from build123d import *

# Parameters (mm, degrees)
SKETCH2_R           = 1.55
CUT_EXTRUDE1_DEPTH  = 33.995567884
SKETCH3_R           = 1.45
BOSS_EXTRUDE1_DEPTH = 1.27
CHAMFER1_SIZE       = 2.54


with BuildPart() as part:
    # Sketch1 → Revolve1 (revolve)
    with BuildSketch(Plane(origin=(0, 0, 0), x_dir=(0, 0, -1), z_dir=(1, 0, 0))):
        Polygon((0, 0), (0, -6.35), (-4.975, -6.35), (-4.975, 0), (-19.05, 0), (-19.05, 12.7), (0, 12.7), align=None)
    revolve(axis=Axis((0, 12.7, 0), (0, -1, 0)))

    # Sketch2 → Cut-Extrude1 (cut, through all)
    with BuildSketch(Plane(origin=(0, 12.7, 0), x_dir=(1, 0, 0), z_dir=(0, 1, 0))):
        with Locations(Location((0, 9, 0), (0, 0, 270))):
            Circle(SKETCH2_R)
        with Locations(Location((0, -9, 0), (0, 0, 270))):
            Circle(SKETCH2_R)
        with Locations(Location((9, 0, 0), (0, 0, 270))):
            Circle(SKETCH2_R)
        with Locations(Location((-9, 0, 0), (0, 0, 270))):
            Circle(SKETCH2_R)
    extrude(amount=-CUT_EXTRUDE1_DEPTH, mode=Mode.SUBTRACT)

    # Sketch3 → Boss-Extrude1 (add)
    with BuildSketch(Plane.XZ):
        with Locations(Location((-5.08, -5.08, 0), (0, 0, 270))):
            Circle(SKETCH3_R)
        with Locations(Location((-5.08, 5.08, 0), (0, 0, 270))):
            Circle(SKETCH3_R)
        with Locations(Location((5.08, 5.08, 0), (0, 0, 270))):
            Circle(SKETCH3_R)
        with Locations(Location((5.08, -5.08, 0), (0, 0, 270))):
            Circle(SKETCH3_R)
    extrude(amount=BOSS_EXTRUDE1_DEPTH)

    # Chamfer1
    chamfer1_edges = [part.edges().sort_by_distance(p)[0] for p in [
        (0, 12.7, -19.05),
    ]]
    chamfer(chamfer1_edges, length=CHAMFER1_SIZE)


solid = part.part
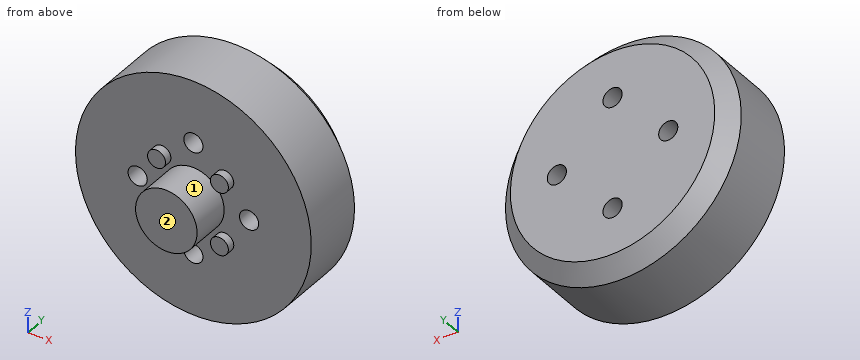
Source: CAD feature listing. Evaluate the final solid. Frame: model axes, mm. Face numbers are marked on the shaded views. A direction names the side the tool comes from. Give positions to 0.01 mm unless a question says otherwise; leave off trailing zeros. Write each loop counter-clockwise with the first axis right and the second up, starting at its lowest first coordinate (ties: lowest second). Pieces come first, ordered by that corner, then holes. Notation, with made-up numbers: (73, 72) -> (117, 72) arc R23 cw to (117, 94) -> close; hole circle Ø6 at (-10, 37). An arc over 180 degrees is marked (long way). Return JSON: item names as keys, results as strings. Group by question number.
1. Section B-B, the plane y = 2. Output: boundary loops of the cut face in (x, z).
2. Section A-A, the plane x = 0. Output: boundary loops of the cut face in (y, z) (3 decimals).
3. Material intervals for line 1 (Z direction, x = 1, y = 7.5); line 2 (Y direction, x = -0.5, z = 10.5); line 3 (X direction, y = 10, z = 8), sorted ascending. Write a range as from..to.
4. Pin query (flat end, axial travel): pin 1 Ø1 at (y, z) = (6, 0.5) entering from +X; pin 2 Ø6 at (y, z) = (5, 0.5) entering from -X; pin 3 Ø5 at (x, y) = (-7, -4) entering from +Z; pin 4 Ø3 at (x, z) = (0, 9) entering from +Y. Return the tip coordinate at first contact, or that it passes through.
5. Access query for the marked faces 1 and 2. Directions: +Z, -Z, +X, -X, +Y, -Y. A direction counts if a zero-diameter tool reaches every point of the face in a straight line with its end or side. Return the directions, or none.
6. Section C-C, the plane z = 0. Output: boundary loops of the cut face in (x, y) (3 decimals), then the cut area to 3 significant figures.
Determined:
{
 "1": {"outline": "circle Ø38.1 at (0, 0); hole circle Ø3.1 at (-9, 0); hole circle Ø3.1 at (0, -9); hole circle Ø3.1 at (0, 9); hole circle Ø3.1 at (9, 0)"},
 "2": {"outline": "(-6.35, -4.975) -> (0, -4.975) -> (0, -7.45) -> (12.7, -7.45) -> (12.7, 7.45) -> (0, 7.45) -> (0, 4.975) -> (-6.35, 4.975) -> close; (0, -19.05) -> (10.16, -19.05) -> (12.7, -16.51) -> (12.7, -10.55) -> (0, -10.55) -> close; (0, 10.55) -> (12.7, 10.55) -> (12.7, 16.51) -> (10.16, 19.05) -> (0, 19.05) -> close"},
 "3": {"line 1": "z = -19.02..-10.18, -7.82..7.82, 10.18..19.02", "line 2": "y = 0..12.7", "line 3": "x = -17.29..-1.18, 1.18..17.29"},
 "4": {"pin 1": "stops at x = 19.05", "pin 2": "stops at x = -19.05", "pin 3": "stops at z = 2.12", "pin 4": "passes through"},
 "5": {"face 1": "-Y", "face 2": "+Z, -Z, +X, -X, -Y"},
 "6": {"outline": "(-19.05, 0) -> (-10.55, 0) -> (-10.55, 12.7) -> (-16.51, 12.7) -> (-19.05, 10.16) -> close; (-7.45, 0) -> (-4.975, 0) -> (-4.975, -6.35) -> (4.975, -6.35) -> (4.975, 0) -> (7.45, 0) -> (7.45, 12.7) -> (-7.45, 12.7) -> close; (10.55, 0) -> (19.05, 0) -> (19.05, 10.16) -> (16.51, 12.7) -> (10.55, 12.7) -> close", "area": "462 mm2"}
}
